from build123d import *

# Parameters (mm, degrees)
SKETCH_1_W          = 8
SKETCH_1_H          = 18
EXTRUDE_1_DEPTH     = 4
CUT_EXTRUDE_4_DEPTH = 1.5
SKETCH_6_W          = 8
SKETCH_6_H          = 1.2
CUT_EXTRUDE_5_DEPTH = 13.68857754
SKETCH_7_R          = 1
CUT_EXTRUDE_6_DEPTH = 11.161200716
FILLET_1_R          = 3
FILLET_2_R          = 2
FILLET_3_R          = 1.5
CUT_EXTRUDE_START   = -4
CUT_EXTRUDE_7_DEPTH = 4


# Read off the part's stored shape, not the designer's step: 切除-拉伸7
with BuildPart() as part:
    # 草图1 → 凸台-拉伸1 (new body)
    with BuildSketch(Plane(origin=(0, 0, 0), x_dir=(1, 0, 0), z_dir=(0, 1, 0))):
        Rectangle(SKETCH_1_W, SKETCH_1_H)
    extrude(amount=EXTRUDE_1_DEPTH)

    # 草图5 → 切除-拉伸4 (cut)
    with BuildSketch(Plane(origin=(0, 4, 0), x_dir=(1, 0, 0), z_dir=(0, 1, 0))):
        with BuildLine():
            Line((2.005613872, -8), (-1.994386128, -8))
            Line((-1.994386128, -8), (-1.994386128, 3.12672716))
            ThreePointArc((-1.994386128, 3.12672716), (-0.007347569, 8.599991292), (2.005613872, 3.136207921))
            Line((2.005613872, 3.136207921), (2.005613872, -8))
        make_face()
    extrude(amount=-CUT_EXTRUDE_4_DEPTH, mode=Mode.SUBTRACT)

    # 草图6 → 切除-拉伸5 (cut, through all)
    with BuildSketch(Plane(origin=(4, 0, 0), x_dir=(0, 0, -1), z_dir=(1, 0, 0))):
        with Locations((-4, 1.5)):
            Rectangle(SKETCH_6_W, SKETCH_6_H)
    extrude(amount=-CUT_EXTRUDE_5_DEPTH, mode=Mode.SUBTRACT)

    # 草图7 → 切除-拉伸6 (cut, through all)
    with BuildSketch(Plane(origin=(0, 2.5, 0), x_dir=(1, 0, 0), z_dir=(0, 1, 0))):
        with Locations(Location((0, 5.5, 0), (0, 0, 270))):
            Circle(SKETCH_7_R)
    extrude(amount=-CUT_EXTRUDE_6_DEPTH, mode=Mode.SUBTRACT)

    # 圆角1
    fillet_1_edges = [part.edges().sort_by_distance(p)[0] for p in [
        (-4, 2, -9),
        (4, 2, -9),
    ]]
    fillet(fillet_1_edges, radius=FILLET_1_R)

    # 圆角2
    # the kernel refuses this fillet: 2 mm, written as the material it takes off along each edge
    with BuildSketch(Plane(origin=(4, -5, 9), x_dir=(0, 0, -1), z_dir=(0, 1, 0)), Plane(origin=(-4, -5, 9), x_dir=(1, 0, 0), z_dir=(0, 1, 0))) as fillet_2_piece_1:
        with BuildLine():
            CenterArc((FILLET_2_R, FILLET_2_R), FILLET_2_R, 180, 90)
            Line((0, FILLET_2_R), (0, 0))
            Line((0, 0), (FILLET_2_R, 0))
        make_face()
    extrude(amount=14, mode=Mode.SUBTRACT)

    # 圆角3
    fillet_3_edges = [part.edges().sort_by_distance(p)[0] for p in [
        (2.005613872, 3.25, 8),
        (-1.994386128, 3.25, 8),
    ]]
    fillet(fillet_3_edges, radius=FILLET_3_R)

    # 切除-拉伸7 outline → 切除-拉伸7 (cut)
    with BuildSketch(Plane(origin=(0, 4, 0), x_dir=(1, 0, 0), z_dir=(0, 1, 0)).offset(CUT_EXTRUDE_START)):
        with BuildLine():
            ThreePointArc((-3.34354323, 7.872913541), (-3.683281573, 7.341640787), (-3.904456771, 6.751086459))
            ThreePointArc((-3.904456771, 6.751086459), (-3.667151483, 7.333575742), (-3.34354323, 7.872913541))
        make_face()
        with BuildLine():
            ThreePointArc((3.34354323, 7.872913541), (3.667151483, 7.333575742), (3.90445677, 6.751086459))
            ThreePointArc((3.90445677, 6.751086459), (3.683281573, 7.341640787), (3.34354323, 7.872913541))
        make_face()
        with BuildLine():
            ThreePointArc((-2.994386128, 2.699347983), (-3.62401419, 3.582574342), (-4, 4.6))
            Line((-4, 4.6), (-4, -7))
            ThreePointArc((-4, -7), (-3.414213562, -8.414213562), (-2, -9))
            Line((-2, -9), (-0.494386128, -9))
            ThreePointArc((-0.494386128, -9), (-2.262153081, -8.267766953), (-2.994386128, -6.5))
            Line((-2.994386128, -6.5), (-2.994386128, 2.699347983))
        make_face()
        with BuildLine():
            Line((4, -7), (4, 4.6))
            ThreePointArc((4, 4.6), (3.627858614, 3.589858153), (3.005613872, 2.711400845))
            Line((3.005613872, 2.711400845), (3.005613872, -6.5))
            ThreePointArc((3.005613872, -6.5), (2.273380825, -8.267766953), (0.505613872, -9))
            Line((0.505613872, -9), (2, -9))
            ThreePointArc((2, -9), (3.414213562, -8.414213562), (4, -7))
        make_face()
    extrude(amount=CUT_EXTRUDE_7_DEPTH, mode=Mode.SUBTRACT)


solid = part.part
Could you check a few things on this model? Use its own coordinates, in mm. A direction names the side the tool comes from. Coordinates: 2 decimals unless noted, no trailing zeros. Order: outer loops, then holes, each group sorted by start corner. A loop starts at its lowest first (then second) coordinate and runs counter-clockwise, first axis right, second up. Notation, with made-up numbers: (80.25, 25) -> (91.25, 25) arc R38 cw to (91.25, 63) -> close; hole circle Ø10 at (63.25, 85). An arc over 180 degrees is marked (long way). One line per question, with ' | ' between items.
Q1. Imagine slicing it at C-C on z = -1.25. Please give me the cut outline in (x, y), and give its area (3 significant figures).
Return value:
outline: (-2.99, 0) -> (3.01, 0) -> (3.01, 4) -> (2.01, 4) -> (2.01, 2.5) -> (-1.99, 2.5) -> (-1.99, 4) -> (-2.99, 4) -> close | area: 18.0 mm²
Q2. Imagine slicing it at D-D on y = 3.55. Please give me the cut outline in (x, z).
Return value:
outline: (-4, -6) arc R3 ccw to (-3.9, -6.75) arc R4.1 ccw to (-3.34, -7.87) arc R3 ccw to (-1, -9) -> (1, -9) arc R3 ccw to (3.34, -7.87) arc R4.1 ccw to (3.9, -6.75) arc R3 ccw to (4, -6) -> (4, -4.6) arc R4.1 ccw to (3.01, -2.71) -> (3.01, 6.5) arc R2.5 ccw to (0.51, 9) -> (-0.49, 9) arc R2.5 ccw to (-2.99, 6.5) -> (-2.99, -2.7) arc R4.1 ccw to (-4, -4.6) -> close; hole (-1.99, -3.13) arc R3.1 ccw (long way) to (2.01, -3.14) -> (2.01, 6.5) arc R1.5 ccw to (0.51, 8) -> (-0.49, 8) arc R1.5 ccw to (-1.99, 6.5) -> close
Q3. Thinking about a two-plate mould opening in Z: for faces 4 (the face through (0, 2, -9)), 5 (the face through (4, 2, -5)), 6 (the face through (-1.543, 3.24, 7.572)), which applies, pulls with the +Z half, pulls with the -Z half, needs draft (parallel to the pull), parting line crosses it, or undercut?
Return value:
face 4: pulls with the -Z half | face 5: needs draft | face 6: undercut
Q4. Imagine slicing it at B-B on y = 1.3. Please give me the cut outline in (x, z), and give its area (3 significant figures).
Return value:
outline: (-4, -6) arc R3 ccw to (-3.9, -6.75) arc R4.1 ccw to (-3.34, -7.87) arc R3 ccw to (-1, -9) -> (1, -9) arc R3 ccw to (3.34, -7.87) arc R4.1 ccw to (3.9, -6.75) arc R3 ccw to (4, -6) -> (4, -4.6) arc R4.1 ccw to (3.01, -2.71) -> (3.01, 0) -> (-2.99, 0) -> (-2.99, -2.7) arc R4.1 ccw to (-4, -4.6) -> close; (-2.49, 8) -> (2.51, 8) arc R2.5 ccw to (0.51, 9) -> (-0.49, 9) arc R2.5 ccw to start; hole circle Ø2 at (0, -5.5) | area: 61.9 mm²
Q5. If I drill on L1, parallel to X at y = 1.75, z = -5.5; L2, parallel to Y at x = 1.75, z = 1; L3, parallel to X at y = 2.75, z = 6.5, over which ranges is the centre line in solid material (lowest first)?
Return value:
L1: -4 to -1, 1 to 4 | L2: 0 to 0.9, 2.1 to 2.5 | L3: -2.99 to -1.99, 2.01 to 3.01
Q6. Imagine slicing it at A-A on z = -5.5. Please give me the cut outline in (x, y).
Return value:
outline: (-4, 0) -> (-1, 0) -> (-1, 2.5) -> (-3.1, 2.5) -> (-3.1, 4) -> (-4, 4) -> close; (1, 0) -> (4, 0) -> (4, 4) -> (3.1, 4) -> (3.1, 2.5) -> (1, 2.5) -> close
Q7. On a 3-axis mill with a long thin cutter (end or side, diameter ignored), from which of +Z, -Z, +X, -X, +Y, -Y can I reach the whole of each face in a straight line? I mean faces 1 (the face through (2.006, 3, 2)), 2 (the face through (0, 2.1, 4)), 3 (the face through (-2.994, 2.4, 2)). Say none if no direction works.
Return value:
face 1: +Y | face 2: +X, -X | face 3: +Z, -X, +Y, -Y
Q8. I'm going to push flat-ended pins straight in: P1, Ø1.8, axis at x = -1, z = 5.5, coming from the +Y side; P2, Ø1.2, axis at x = 0, z = -5.5, coming from the -Y side; P3, Ø0.8, axis at y = 3, z = -0.5, coming from the +X side; P4, Ø2, axis at y = 2, z = 1, coming from the -X side. Where does each tip first touch, or does it pass through?
Return value:
P1: y = 2.5 | P2: through | P3: x = 3.01 | P4: x = -2.99
